```python
from build123d import *

# Parameters (mm, degrees)
SKETCH1_W                   = 25.4
SKETCH1_H                   = 69.85
BOSS_EXTRUDE1_DEPTH         = 162.56
SKETCH2_R                   = 4.7625
CUT_EXTRUDE1_DEPTH          = 50.8
SKETCH3_W                   = 7.62
SKETCH3_H                   = 76.2
CUT_EXTRUDE2_DEPTH          = 179.745450571
SKETCH4_W                   = 25.4
SKETCH4_H                   = 12.7
CUT_EXTRUDE3_DEPTH          = 179.745450571
F_1_4_20_TAPPED_HOLE1_D     = 5.1054
F_1_4_20_TAPPED_HOLE1_DEPTH = 22.86
F_1_4_20_TAPPED_HOLE1_TIP   = 1.533816902


with BuildPart() as part:
    # Sketch1 → Boss-Extrude1 (new body)
    with BuildSketch(Plane(origin=(0, 0, 0), x_dir=(1, 0, 0), z_dir=(0, 1, 0))):
        with Locations((12.7, 34.925)):
            Rectangle(SKETCH1_W, SKETCH1_H)
    extrude(amount=BOSS_EXTRUDE1_DEPTH)

    # Sketch2 → Cut-Extrude1 (cut)
    with BuildSketch(Plane(origin=(0, 162.56, 0), x_dir=(1, 0, 0), z_dir=(0, 1, 0))):
        with Locations(Location((12.7, 25.4, 0), (0, 0, 270))):
            Circle(SKETCH2_R)
    extrude(amount=-CUT_EXTRUDE1_DEPTH, mode=Mode.SUBTRACT)

    # Sketch3 → Cut-Extrude2 (cut, through all)
    with BuildSketch(Plane.XY):
        with Locations((3.81, 38.1)):
            Rectangle(SKETCH3_W, SKETCH3_H)
    extrude(amount=-CUT_EXTRUDE2_DEPTH, mode=Mode.SUBTRACT)

    # Sketch4 → Cut-Extrude3 (cut, through all)
    with BuildSketch(Plane(origin=(25.4, 0, 0), x_dir=(0, 0, -1), z_dir=(1, 0, 0))):
        with Locations((57.15, 156.21)):
            Rectangle(SKETCH4_W, SKETCH4_H)
    extrude(amount=-CUT_EXTRUDE3_DEPTH, mode=Mode.SUBTRACT)

    # 1/4-20 Tapped Hole1
    with Locations(Plane(origin=(0, 0, -69.85), x_dir=(-1, 0, 0), z_dir=(0, 0, -1))):
        with Locations((-17.78, 43.18), (-17.78, 12.7)):
            Hole(F_1_4_20_TAPPED_HOLE1_D / 2, depth=F_1_4_20_TAPPED_HOLE1_DEPTH)
            with Locations((0, 0, -(F_1_4_20_TAPPED_HOLE1_DEPTH + F_1_4_20_TAPPED_HOLE1_TIP / 2))):  # 118° drill point
                Cone(0, F_1_4_20_TAPPED_HOLE1_D / 2, F_1_4_20_TAPPED_HOLE1_TIP, mode=Mode.SUBTRACT)


solid = part.part
```
The listing builds one solid part. Answer for the finished solid, in the listing's coordinates (mm). A direction names the side the tool comes from. Coordinates: 2 decimals unless noted, no trailing zeros. Order: outer loops, then holes, each group sorted by start corner. A loop starts at its lowest first (then second) coordinate and runs counter-clockwise, first axis right, second up. Notation, with made-up numbers: M 27.5,39 L 64.5,39 A24 ccw 64.5,68 Z; hole C 84.25,89 d2. An arc over 180 degrees is marked long. Answer as a JSON object with one key per item and string values. Group by question number.
1. Determine the mould class of faces 1 (the conical face through (17.838, 13.14, -45.723)), 2 (the flat face through (0, 119, -34)), 3 (the flat face through (13, 156, -44.45)), 4 (the cylindrical face through (15.75, 11.15, -58.26)) for opening direction X: released by +X, released by -X, zero draft, split by the parting line, or undercut.
2. Section D-D on z = -25.4 is taken. Write down the section's boundary in (x, y).
3. A tool of negligible diameter and unlimited length cuts with its end or side. For faces 5 (the cylindrical face through (17.227, 40.688, -58.26)), 6 (the cylindrical face through (10.88, 137.52, -21)), 7 (the flat face through (13, 149.86, -57)), from which of +Z, -Z, +X, -X, +Y, -Y can it reach the whole face along a straight path? Write none if from no direction.
4. Flat-ended cylindrical pins translate along their axes: P1, Ø21, axis at y = 34, z = -32, coming from the -X side; P2, Ø6.5, axis at x = 17.78, y = 12.7, coming from the -Z side; P3, Ø6.5, axis at x = 14.5, y = 154.5, coming from the -Z side; P4, Ø4, axis at x = 4.5, z = -29, coming from the -Y side. Find the tip coordinate at first contact, or state that the pin passes through.
5. Section C-C on z = -33 is taken. Write down the section's boundary in (x, y), then the cut area to 3 significant figures.
6. Straight lines are drawn through the part: line 1 (Y direction, x = 17.78, z = -53); line 2 (X direction, y = 12.7, z = -61); line 3 (X direction, y = 135.5, z = -25.4). For each, find the intervals that lie inside material, in ascending order.
7. Section B-B on x = 12.7 is taken. Write down the section's boundary in (y, z), then the cut area to 3 significant figures.
Values follow:
{
 "1": {"face 1": "undercut", "face 2": "released by -X", "face 3": "zero draft", "face 4": "undercut"},
 "2": {"outline": "M 0,76.2 L 7.62,76.2 L 7.62,0 L 25.4,0 L 25.4,162.56 L 17.46,162.56 L 17.46,111.76 L 7.94,111.76 L 7.94,162.56 L 0,162.56 Z"},
 "3": {"face 5": "-Z", "face 6": "+Y", "face 7": "-Z, +X, -X, +Y"},
 "4": {"P1": "x = 7.62", "P2": "z = -69.85", "P3": "z = -44.45", "P4": "y = 76.2"},
 "5": {"outline": "M 0,76.2 L 7.62,76.2 L 7.62,0 L 25.4,0 L 25.4,162.56 L 0,162.56 Z", "area": "3,550 mm2"},
 "6": {"line 1": "0 to 10.15, 15.25 to 40.63, 45.73 to 149.86", "line 2": "7.62 to 15.23, 20.33 to 25.4", "line 3": "0 to 7.94, 17.46 to 25.4"},
 "7": {"outline": "M 0,-69.85 L 149.86,-69.85 L 149.86,-44.45 L 162.56,-44.45 L 162.56,-30.16 L 111.76,-30.16 L 111.76,-20.64 L 162.56,-20.64 L 162.56,0 L 0,0 Z", "area": "10,500 mm2"}
}
